Geometry check sheet. Reference: the model listing, model coordinates, mm. A direction names the side the tool comes from. Give positions to 0.01 mm unless a question says otherwise; leave off trailing zeros. Loops run counter-clockwise (first coordinate to the right, second up) from the corner with the lowest first, then second, coordinate; pieces in that order, holes last. Notation, with made-up numbers: (76, 45) -> (115, 45) arc R33 ccw to (115, 75) -> close; hole circle Ø3 at (-37, 37). An arc over 180 degrees is marked (long way). Answer as a JSON object with one key per item and string values.
from build123d import *

# Parameters (mm, degrees)
SKETCH_1_R               = 5
EXTRUDE_1_DEPTH          = 40
CUT_EXTRUDE_1_DEPTH      = 18
CUT_EXTRUDE_1_DEPTH_BACK = 18
SKETCH_2_W               = 81.294716022
SKETCH_2_H               = 74
SKETCH_3_R               = 4
EXTRUDE_2_DEPTH          = 25
SKETCH_4_W               = 2
SKETCH_4_H               = 40
EXTRUDE_3_DEPTH          = 42


with BuildPart() as part:
    # 草图1 → 凸台-拉伸1 (new body)
    with BuildSketch(Plane.XY):
        with BuildLine():
            Line((0, 39), (-40, 39))
            Line((-40, 39), (-15, 0))
            ThreePointArc((-15, 0), (0, -15), (15, 0))
            Line((15, 0), (40, 39))
            Line((40, 39), (0, 39))
        make_face()
        Circle(SKETCH_1_R, mode=Mode.SUBTRACT)
    extrude(amount=EXTRUDE_1_DEPTH)

    # 草图2 → 切除-拉伸1 (cut, two sides: drawn at the far end of the back side and taken through both)
    with BuildSketch(Plane.XY.offset(20).offset(-CUT_EXTRUDE_1_DEPTH_BACK)):
        Rectangle(SKETCH_2_W, SKETCH_2_H)
    extrude(amount=CUT_EXTRUDE_1_DEPTH + CUT_EXTRUDE_1_DEPTH_BACK, mode=Mode.SUBTRACT)

    # 草图3 → 凸台-拉伸2 (add)
    with BuildSketch(Plane(origin=(0, 39, 0), x_dir=(1, 0, 0), z_dir=(0, 1, 0))):
        with Locations((0, -20)):
            Circle(SKETCH_3_R)
    extrude(amount=EXTRUDE_2_DEPTH)

    # 草图4 → 凸台-拉伸3 (add)
    with BuildSketch(Plane(origin=(0, 39, 0), x_dir=(1, 0, 0), z_dir=(0, 1, 0))):
        with Locations((39, -20)):
            Rectangle(SKETCH_4_W, SKETCH_4_H)
    extrude(amount=-EXTRUDE_3_DEPTH)


solid = part.part
1) Draft check along Y on faces 5 (the face through (0, -15, 39)), 6 (the face through (0.6, 39, 24.2)), 7 (the face through (-1.08, -4.88, 0.99)). Enter one of: pulls with the +Y half, pulls with the -Y half, needs draft (parallel to the pull), parting line crosses it, or undercut.
Geometry check:
{"face 5": "pulls with the -Y half", "face 6": "pulls with the +Y half", "face 7": "undercut"}
2) Section check B-B on y = 32.5. Record the cut outline in (x, z).
Geometry check:
{"outline": "(-35.83, 0) -> (35.83, 0) -> (35.83, 2) -> (-35.83, 2) -> close; (-35.83, 38) -> (35.83, 38) -> (35.83, 40) -> (-35.83, 40) -> close; (38, 0) -> (40, 0) -> (40, 40) -> (38, 40) -> close"}
3) Material ranges on line 1 along X through (y, z) = (0, 38.6); line 2 along Z through (x, y) = (-27, 35); line 3 along Y through (x, z) = (0, 1.15), recorded low to high. Write a range as from..to.
Geometry check:
{"line 1": "x = -15..-5, 5..15, 38..40", "line 2": "z = 0..2, 38..40", "line 3": "y = -15..-5, 5..39"}
4) Section check C-C on z = 20. Record the cut outline in (x, y).
Geometry check:
{"outline": "(-40, 39) -> (-38.72, 37) -> (38, 37) -> (38, -3) -> (40, -3) -> (40, 39) -> (4, 39) -> (4, 64) -> (-4, 64) -> (-4, 39) -> close"}
5) Section check A-A on x = 0. Record the cut outline in (y, z).
Geometry check:
{"outline": "(-15, 0) -> (-5, 0) -> (-5, 2) -> (-15, 2) -> close; (-15, 38) -> (-5, 38) -> (-5, 40) -> (-15, 40) -> close; (5, 0) -> (39, 0) -> (39, 16) -> (64, 16) -> (64, 24) -> (39, 24) -> (39, 40) -> (5, 40) -> (5, 38) -> (37, 38) -> (37, 2) -> (5, 2) -> close"}
6) Section check D-D on x = -19. Record the cut outline in (y, z).
Geometry check:
{"outline": "(6.24, 0) -> (39, 0) -> (39, 40) -> (6.24, 40) -> (6.24, 38) -> (37, 38) -> (37, 2) -> (6.24, 2) -> close"}
7) Tool access check on faces 1 (the face through (-0.521, 51.325, 16.034)), 2 (the face through (26.34, 17.69, 38.99)), 3 (the face through (-39.595, 38.369, 19.907)), 4 (the face through (-1, 37, 20)). Record the directions out of +Z, -Z, +X, -X, +Y, -Y that give a thin tool (end or side, any length) a straight path to the whole face; none if there is none.
Geometry check:
{"face 1": "+Y", "face 2": "+Z, -Z, -Y", "face 3": "+Z, -Z, -X, -Y", "face 4": "-X, -Y"}
8) Depth check by flat-ended pin: P1, Ø6, axis at x = -11, z = 32.5, coming from the -Y side; P2, Ø2, axis at x = 39, z = 14, coming from the -Y side; P3, Ø6, axis at x = -7.5, z = 4.5, coming from the +Y side. Enter the tip coordinate at first touch or a pass-through.
Geometry check:
{"P1": "stops at y = 37", "P2": "stops at y = -3", "P3": "stops at y = 39"}
